Job drawing, mm, ordinate dimensions from the low corner. One solid piece. Give positions to 0.01 mm unless a question says otherwise; leave off trailing zeros. Write each loop counter-clockwise with the first axis right and the second up, starting at its lowest first coordinate (ties: lowest second). Pieces come first, ordered by that corner, then holes. Notation, with made-up numbers: (-35.75, 27.5) - (-20.75, 27.5) arc R19 ccw to (-20.75, 63.5) - close; hole circle Ø9 at (5, 70). An arc over 180 degrees is marked (long way). Use a Markdown table: item, result. Add a question column.
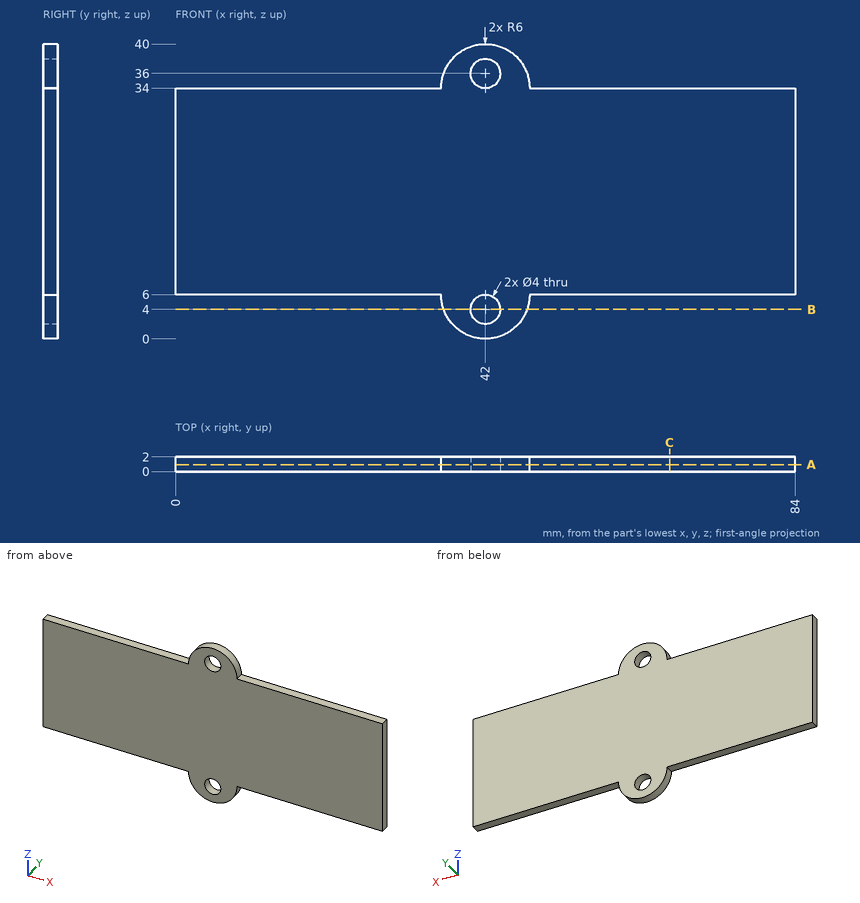
(1) Band-saw the part on A-A (y = 0.95). Write the cut outline in (x, z).
(2) Band-saw the part on B-B (z = 4). Write the cut outline in (x, y).
(3) Band-saw the part on C-C (x = 67). Write the cut outline in (y, z), then the cut area to 3 significant figures.
(4) Flat gauge pins, fed straight in: pin 1 (1 mm diameter, centred on x = 23.5, y = 0.5, fed in from -Z); pin 2 (1 mm diameter, centred on x = 37, y = 0.5, fed in from -Z); pin 3 (3.5 mm diameter, centred on x = 42, z = 36, fed in from +Y); pin 4 (5 mm diameter, centred on x = 42, z = 4, fed in from +Y). Where does each tip first touch, or does it go through?
(5) Probe probe 1 along X at (y, z) = (1.5, 36); probe 2 along Z at (x, y) = (15, 0.7); probe 3 along X at (y, z) = (1.25, 35). List the from-to ranges inside material, lowest first. Write a range as [from, to].
Model answer:
| question | item | result |
|---|---|---|
| 1 | outline | (0, 6) - (36, 6) arc R6 ccw to (48, 6) - (84, 6) - (84, 34) - (48, 34) arc R6 ccw to (36, 34) - (0, 34) - close; hole circle Ø4 at (42, 4); hole circle Ø4 at (42, 36) |
| 2 | outline | (36.34, 0) - (40, 0) - (40, 2) - (36.34, 2) - close; (44, 0) - (47.66, 0) - (47.66, 2) - (44, 2) - close |
| 3 | outline | (0, 6) - (2, 6) - (2, 34) - (0, 34) - close |
| 3 | area | 56.0 mm^2 |
| 4 | pin 1 | stops at z = 6 |
| 4 | pin 2 | stops at z = 2.03 |
| 4 | pin 3 | passes through |
| 4 | pin 4 | stops at y = 2 |
| 5 | probe 1 | x = [36.34, 40], [44, 47.66] |
| 5 | probe 2 | z = [6, 34] |
| 5 | probe 3 | x = [36.08, 40.27], [43.73, 47.92] |
